Design review of the part shown in the three views and the two pictorial views. Dimensions are in mm from the part's minimum x, y and z. Round coordinates to 2 decimals unless told otherwise and drop trailing zeros. Loops run counter-clockwise (first coordinate to the right, second up) from the corner with the lowest first, then second, coordinate; pieces in that order, holes last.
1) Insertion check: pin 1 (3 mm diameter, centred on x = 15, z = 45.5, fed in from -Y). The pin has a flat end and moves straight along its axis. Give the tip position at first contact, or say it passes through.
2) Take a section at B-B (x = 25). State the section outline as (y, z) points.
3) Take a section at C-C (z = 84.5). State the section outline as (x, y) points, then the cut area to 3 significant figures.
4) Wall thickness on L1, parallel to X at y = 1.45, z = 21; L2, parallel to Z at x = 79.5, y = 1.2; L3, parallel to Z at x = 51, y = 1: over which ranges is each line inside the solid? List them lowest first.
5) Take a section at A-A (y = 0.3). State the section outline as (x, z) points, then the cut area to 3 significant figures.
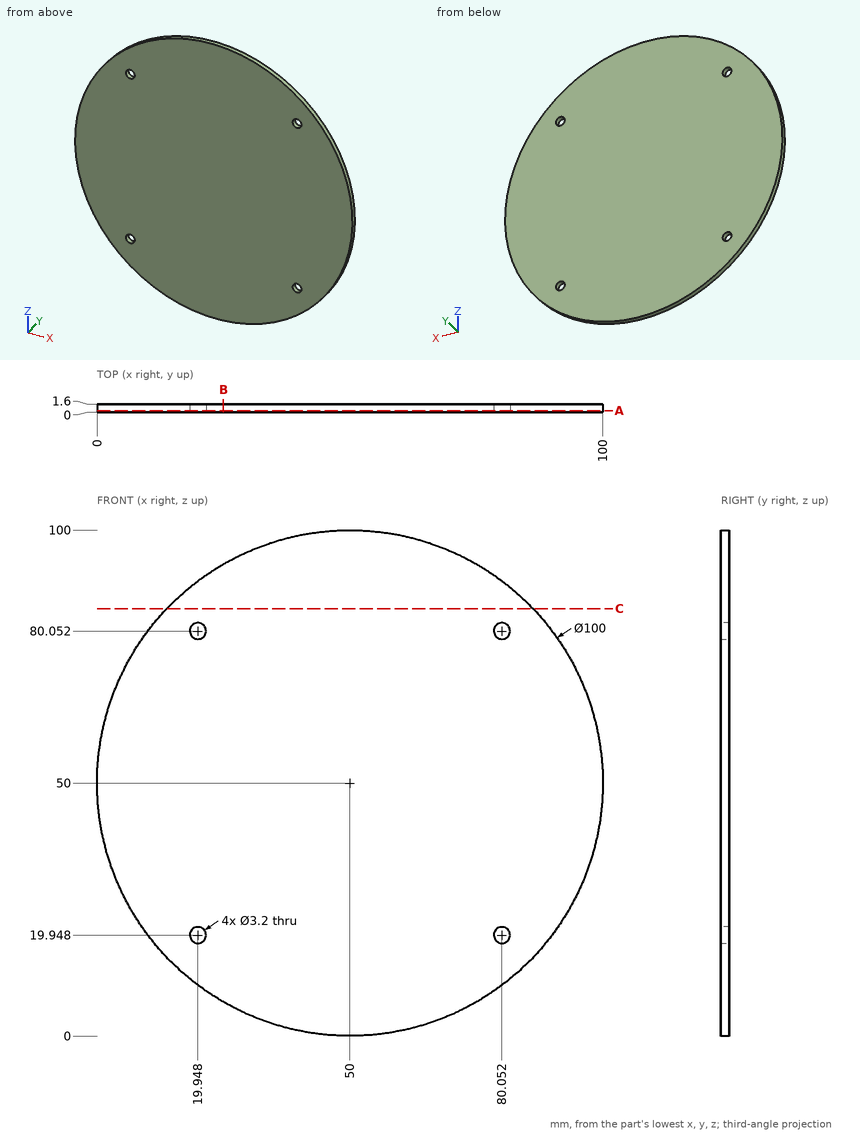
Response:
1. pin 1: stops at y = 0
2. outline: (0, 6.7) - (1.6, 6.7) - (1.6, 93.3) - (0, 93.3) - close
3. outline: (13.81, 0) - (86.19, 0) - (86.19, 1.6) - (13.81, 1.6) - close
3. area: 116 mm2
4. L1: x = 9.27 to 18.74, 21.15 to 78.85, 81.26 to 90.73
4. L2: z = 9.63 to 18.45, 21.45 to 78.55, 81.55 to 90.37
4. L3: z = 0.01 to 99.99
5. outline: circle Ø100 at (50, 50); hole circle Ø3.2 at (19.95, 19.95); hole circle Ø3.2 at (19.95, 80.05); hole circle Ø3.2 at (80.05, 19.95); hole circle Ø3.2 at (80.05, 80.05)
5. area: 7,820 mm2
